Autodesk Inventor part; units mm, degrees
ref_plane "YZ Plane" through (0, 0, 0) normal (1, 0, 0) x (0, 1, 0)
ref_plane "XZ Plane" through (0, 0, 0) normal (0, 1, 0) x (-1, 0, 0)
ref_plane "XY Plane" through (0, 0, 0) normal (0, 0, 1) x (1, 0, 0)
sketch "Эскиз1" plane through (0, 0, 0) normal (0, 0, 1) x (1, 0, 0)
  line L0 (-32.5, -22.5) -> (-32.5, -19.5)
  line L1 (-32.5, -19.5) -> (-42.5, -19.5)
  line L2 (-42.5, -19.5) -> (-42.5, -22.5)
  line L3 (0, -19.5) -> (-5, -19.5)
  line L4 (-5, -19.5) -> (-5, -22.5)
  line L5 (-75, 22.5) -> (-42.5, 22.5)
  line L6 (-32.5, 22.5) -> (-32.5, 19.5)
  line L7 (-32.5, 19.5) -> (-42.5, 19.5)
  line L8 (-42.5, 19.5) -> (-42.5, 22.5)
  line L9 (-32.5, 22.5) -> (-5, 22.5)
  line L10 (0, 19.5) -> (-5, 19.5)
  line L11 (-5, 19.5) -> (-5, 22.5)
  line L12 (-5, 22.5) -> (-32.5, 22.5)
  line L13 (-42.5, 22.5) -> (-75, 22.5)
  line L14 (32.5, -22.5) -> (32.5, -19.5)
  line L15 (32.5, -19.5) -> (42.5, -19.5)
  line L16 (42.5, -19.5) -> (42.5, -22.5)
  line L17 (0, -19.5) -> (5, -19.5)
  line L18 (5, -19.5) -> (5, -22.5)
  line L19 (75, 22.5) -> (42.5, 22.5)
  line L20 (32.5, 22.5) -> (32.5, 19.5)
  line L21 (32.5, 19.5) -> (42.5, 19.5)
  line L22 (42.5, 19.5) -> (42.5, 22.5)
  line L23 (32.5, 22.5) -> (5, 22.5)
  line L24 (0, 19.5) -> (5, 19.5)
  line L25 (5, 19.5) -> (5, 22.5)
  line L26 (5, 22.5) -> (32.5, 22.5)
  line L27 (42.5, 22.5) -> (75, 22.5)
  line L28 (-42.5, -22.5) -> (-32.5, -22.5)
  line L29 (-5, -22.5) -> (5, -22.5)
  line L30 (32.5, -22.5) -> (42.5, -22.5)
  line L31 (-32.5, -32.5) -> (-32.5, -29.5)
  line L32 (-32.5, -29.5) -> (-42.5, -29.5)
  line L33 (-42.5, -29.5) -> (-42.5, -32.5)
  line L34 (5, -32.5) -> (5, -29.5)
  line L35 (5, -29.5) -> (-5, -29.5)
  line L36 (-5, -29.5) -> (-5, -32.5)
  line L37 (42.5, -32.5) -> (42.5, -29.5)
  line L38 (42.5, -29.5) -> (32.5, -29.5)
  line L39 (32.5, -29.5) -> (32.5, -32.5)
  line L40 (-75, 2.5) -> (-78, 2.5)
  line L41 (-78, 2.5) -> (-78, -12.5)
  line L42 (-78, -12.5) -> (-75, -12.5)
  line L43 (77.5, 2.5) -> (75, 2.5)
  line L44 (75, -12.5) -> (77.5, -12.5)
  line L45 (77.5, -12.5) -> (77.5, 2.5)
  line L46 (75, -32.5) -> (42.5, -32.5)
  line L47 (32.5, -32.5) -> (5, -32.5)
  line L48 (-5, -32.5) -> (-32.5, -32.5)
  line L49 (-42.5, -32.5) -> (-75, -32.5)
  line L50 (-75, 22.5) -> (-75, 2.5)
  line L51 (-75, -12.5) -> (-75, -32.5)
  line L52 (75, 22.5) -> (75, 2.5)
  line L53 (75, -12.5) -> (75, -32.5)
  point P0 (0, 0)
extrude "Выдавливание2" add sketch "Эскиз1" along normal blind 3
sketch "Эскиз2" plane through (0, 0, 3) normal (0, 0, 1) x (1, 0, 0)
  point P0 (0, 0)
properties part number "Стенка t1"
The model under review builds one solid part; all positions refer to its coordinate system, in mm. A direction names the side the tool comes from. Round coordinates to 2 decimals unless told otherwise and drop trailing zeros. Order: outer loops, then holes, each group sorted by start corner. A loop starts at its lowest first (then second) coordinate and runs counter-clockwise, first axis right, second up. Notation, with made-up numbers: (7, -34) -> (55, -34) arc R19 cw to (55, -30) -> close; hole circle Ø1 at (-40, 55.5). An arc over 180 degrees is marked (long way). Use CSV: the item, a comma, the result in double quotes. Start each with the question number.
(1) Insertion check: pin 1 (0.9 mm diameter, centred on y = 21.5, z = 1.5, fed in from -X); pin 2 (0.9 mm diameter, centred on y = 21, z = 2, fed in from +X); pin 3 (0.9 mm diameter, centred on x = 36.5, z = 2, fed in from -Y). Each pin has a flat end and moves straight along its axis. Give the tip position at first contact, or say it passes through.
(2) Wall thickness on probe 1 along X at (y, z) = (-30, 0.75); probe 2 along Y at (x, z) = (41, 1.5); probe 3 along X at (y, z) = (-27.5, 2.45): over which ranges is each line inside the solid? List them lowest first. Write a range as from..to.
(3) Tool access review of faces 5 (the face through (-37, -19.5, 1)), 6 (the face through (-37, -29.5, 1)), 7 (the face through (5, 21, 1)), 8 (the face through (-77, -12.5, 1)): name each direction out of +Z, -Z, +X, -X, +Y, -Y from which nothing blocks a thin tool from reaching the whole face with its end or side.
(4) Consider section A-A on x = 36. Write out the cut boundary in (y, z).
(5) Consider section C-C on y = 10. Write out the cut boundary in (x, z), and give its area (3 significant figures).
(6) Consider section B-B on z = 1.7. State how many separate pieces and enclosed holes the cut face has, and give its area (3 significant figures).
(7) Mouldability with a two-part tool opening along X and no side actions: class faces 1 (the face through (-42.5, -21, 1)), 2 (the face through (0, -22.5, 1)), 3 (the face through (-75, 13, 1)), 4 (the face through (-59, 22.5, 1)) as pulls with the +X half, pulls with the -X half, needs draft (parallel to the pull), parting line crosses it, or undercut.
Responses:
1,pin 1,"x = -75"
1,pin 2,"x = 75"
1,pin 3,"y = -29.5"
2,probe 1,"-75..-42.5, -32.5..-5, 5..32.5, 42.5..75"
2,probe 2,"-29.5..-22.5, -19.5..19.5"
2,probe 3,"-75..75"
3,face 5,"+Z, -Z"
3,face 6,"+Z, -Z, -Y"
3,face 7,"+Z, -Z, +Y"
3,face 8,"+Z, -Z, -X, -Y"
4,outline,"(-29.5, 0) -> (-22.5, 0) -> (-22.5, 3) -> (-29.5, 3) -> close; (-19.5, 0) -> (19.5, 0) -> (19.5, 3) -> (-19.5, 3) -> close"
5,outline,"(-75, 0) -> (75, 0) -> (75, 3) -> (-75, 3) -> close"
5,area,"450 mm²"
6,separate pieces,"1"
6,enclosed holes,"3"
6,area,"8,060 mm²"
7,face 1,"undercut"
7,face 2,"undercut"
7,face 3,"pulls with the -X half"
7,face 4,"needs draft"
